Build history of the part. All positions in model axes, mm. A direction names the side the tool comes from. Round coordinates to 2 decimals unless told otherwise and drop trailing zeros. Write each loop counter-clockwise with the first axis right and the second up, starting at its lowest first coordinate (ties: lowest second). Pieces come first, ordered by that corner, then holes. Notation, with made-up numbers: (29.25, 43.5) - (57.25, 43.5) arc R12 cw to (57.25, 64.5) - close; hole circle Ø11 at (25, 61). An arc over 180 degrees is marked (long way). Write each question's results on one line, items separated by ' | '.
from build123d import *

# Parameters (mm, degrees)
F2_R     = 11
F2_R_2   = 8.5
F4_DEPTH = 0.5
F0_R     = 11
F0_R_2   = 8.5
F5_R     = 11
F5_R_2   = 10.25
F6_DEPTH = 2.6364565


with BuildPart() as f4:
    # F2 (on offset) → F4 (new body, symmetric)
    with BuildSketch(Plane.XY.offset(6.24)):
        Circle(F2_R)
        Circle(F2_R_2, mode=Mode.SUBTRACT)
    extrude(amount=F4_DEPTH, both=True)



with BuildPart() as f4b:
    # F0 (on Top) → F4, piece 2 (new body, symmetric)
    with BuildSketch(Plane.XY):
        Circle(F0_R)
        Circle(F0_R_2, mode=Mode.SUBTRACT)
    extrude(amount=F4_DEPTH, both=True)


with BuildPart() as f4_1:
    add(f4.part)

    add(f4b.part)  # F6 merges F4b
    # F5 (on offset) → F6 (join, symmetric)
    with BuildSketch(Plane.XY.offset(3.1183971)):
        Circle(F5_R)
        Circle(F5_R_2, mode=Mode.SUBTRACT)
    extrude(amount=F6_DEPTH, both=True)


solid = f4_1.part
(1) Drill centre lines: probe 1 along Y at (x, z) = (0, 6.05); probe 2 along Y at (x, z) = (0, 1.7); probe 3 along Z at (x, y) = (-10, -1.25). Where is each one in solid material? Low to high. Write a range as [from, to].
Worked answers:
probe 1: y = [-11, -8.5], [8.5, 11] | probe 2: y = [-11, -10.25], [10.25, 11] | probe 3: z = [-0.5, 0.5], [5.74, 6.74]
(2) Slice it at A-A, the plane y = 0. Write the cut outline in (x, z), and give its area (3 significant figures).
Worked answers:
outline: (-11, -0.5) - (-8.5, -0.5) - (-8.5, 0.5) - (-10.25, 0.5) - (-10.25, 5.74) - (-8.5, 5.74) - (-8.5, 6.74) - (-11, 6.74) - close; (8.5, -0.5) - (11, -0.5) - (11, 6.74) - (8.5, 6.74) - (8.5, 5.74) - (10.25, 5.74) - (10.25, 0.5) - (8.5, 0.5) - close | area: 17.9 mm2
(3) Slice it at C-C, the plane z = 3.5. Write the cut outline in (x, y), and give its area (3 significant figures).
Worked answers:
outline: circle Ø22 at (0, 0); hole circle Ø20.5 at (0, 0) | area: 50.1 mm2
(4) Two-plate mould, pull along Y, no slides. Class faces 1 (the flat face through (3.2, -8.1, 6.74)), 2 (the cylindrical face through (-2.38, -10.74, 3.17)), 3 (the flat face through (-4, 8, 0.5)): released by +Y, released by -Y, zero draft, split by the parting line, or undercut.
Worked answers:
face 1: zero draft | face 2: split by the parting line | face 3: undercut
(5) Tool access for faces 4 (the flat face through (-4, 8, 5.74)), 5 (the flat face through (3.2, -8.1, -0.5)): list every direction of +Z, -Z, +X, -X, +Y, -Y with a clear straight run to the whole face (end or side of a thin tool).
Worked answers:
face 4: none | face 5: -Z, +X, -X, +Y, -Y
(6) Slice it at D-D, the plane z = 0. Write the cut outline in (x, y).
Worked answers:
outline: circle Ø22 at (0, 0); hole circle Ø17 at (0, 0)
(7) Flat gauge pins, fed straight in: pin 1 Ø2 at (x, z) = (-5, 3.5) entering from +Y; pin 2 Ø10 at (x, y) = (2, -0.5) entering from +Z; pin 3 Ø4 at (x, z) = (4.5, 5.5) entering from +Y. Where does each tip first touch, or does it go through?
Worked answers:
pin 1: stops at y = 10.25 | pin 2: passes through | pin 3: stops at y = 10.71
